```python
from build123d import *

# Parameters (mm, degrees)
SKETCH1_R           = 4.5
BOSS_EXTRUDE1_DEPTH = 5.5
SKETCH2_R           = 4.5
BOSS_EXTRUDE2_DEPTH = 6
SKETCH3_R           = 3
CUT_EXTRUDE1_DEPTH  = 5


with BuildPart() as part:
    # Sketch1 → Boss-Extrude1 (new body)
    with BuildSketch(Plane(origin=(0, 0, 0), x_dir=(1, 0, 0), z_dir=(0, 1, 0))):
        with Locations((-2.5, -1.5)):
            Circle(SKETCH1_R)
        with BuildLine():
            Line((-0.5, 0), (-4.5, 0))
            ThreePointArc((-4.5, 0), (-4.853553391, -0.146446609), (-5, -0.5))
            Line((-5, -0.5), (-5, -2.5))
            ThreePointArc((-5, -2.5), (-4.853553391, -2.853553391), (-4.5, -3))
            Line((-4.5, -3), (-0.5, -3))
            ThreePointArc((-0.5, -3), (-0.146446609, -2.853553391), (0, -2.5))
            Line((0, -2.5), (0, -0.5))
            ThreePointArc((0, -0.5), (-0.146446609, -0.146446609), (-0.5, 0))
        make_face(mode=Mode.SUBTRACT)
    extrude(amount=BOSS_EXTRUDE1_DEPTH)

    # Sketch2 → Boss-Extrude2 (add)
    with BuildSketch(Plane(origin=(0, 5.5, 0), x_dir=(1, 0, 0), z_dir=(0, 1, 0))):
        with Locations((-2.5, -1.5)):
            Circle(SKETCH2_R)
    extrude(amount=BOSS_EXTRUDE2_DEPTH)

    # Sketch3 → Cut-Extrude1 (cut)
    with BuildSketch(Plane(origin=(0, 11.5, 0), x_dir=(1, 0, 0), z_dir=(0, 1, 0))):
        with Locations((-2.5, -1.5)):
            Circle(SKETCH3_R)
    extrude(amount=-CUT_EXTRUDE1_DEPTH, mode=Mode.SUBTRACT)


solid = part.part
```
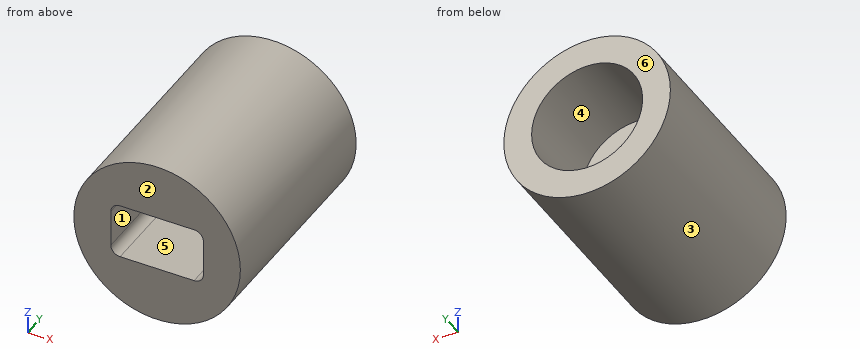
CAD build for the part. Positions are in the model's coordinates, mm. Face numbers are marked on the shaded views. A direction names the side the tool comes from. Round coordinates to 2 decimals unless told otherwise and drop trailing zeros. Write each loop counter-clockwise with the first axis right and the second up, starting at its lowest first coordinate (ties: lowest second). Pieces come first, ordered by that corner, then holes.
Item 1: Mould opens along Z. For the marked faces 1, 2 and 3 say: released by +Z, released by -Z, zero draft, split by the parting line, or undercut.
Filled in:
face 1: undercut
face 2: zero draft
face 3: split by the parting line
Item 2: Tool access for the marked faces 4, 5 and 6: list every direction of +Z, -Z, +X, -X, +Y, -Y with a clear straight run to the whole face (end or side of a thin tool).
Filled in:
face 4: +Y
face 5: -Y
face 6: +Z, -Z, +X, -X, +Y
Item 3: Band-saw the part on C-C on x = -2.5. Write the cut outline in (y, z), then the cut area to 3 significant figures.
Filled in:
outline: (0, -3) - (11.5, -3) - (11.5, -1.5) - (6.5, -1.5) - (6.5, 4.5) - (11.5, 4.5) - (11.5, 6) - (0, 6) - (0, 3) - (5.5, 3) - (5.5, 0) - (0, 0) - close
area: 57.0 mm2
Item 4: Band-saw the part on A-A on y = 1.25. Write the cut outline in (x, z), then the cut area to 3 significant figures.
Filled in:
outline: circle Ø9 at (-2.5, 1.5); hole (-5, 0.5) arc R0.5 ccw to (-4.5, 0) - (-0.5, 0) arc R0.5 ccw to (0, 0.5) - (0, 2.5) arc R0.5 ccw to (-0.5, 3) - (-4.5, 3) arc R0.5 ccw to (-5, 2.5) - close
area: 48.8 mm2
Item 5: Drill centre lines: L1, parallel to Z at x = -2.5, y = 7.65; L2, parallel to X at y = 7.5, z = 1.5; L3, parallel to Z at x = -2.5, y = 1.25. Where is each one in solid material? Low to high.
Filled in:
L1: z = -3 to -1.5, 4.5 to 6
L2: x = -7 to -5.5, 0.5 to 2
L3: z = -3 to 0, 3 to 6
Item 6: Drop flat-ended pins along their axis: pin 1 Ø1.5 at (x, z) = (-2.5, 1) entering from -Y; pin 2 Ø1.5 at (y, z) = (6.5, -1) entering from -X; pin 3 Ø4 at (x, y) = (0.5, 2) entering from -Z; pin 4 Ø2 at (x, y) = (-1.5, 7.5) entering from -Z. Give the stop position or say it passes through.
Filled in:
pin 1: stops at y = 5.5
pin 2: stops at x = -6.65
pin 3: stops at z = -2.89
pin 4: stops at z = -3
Item 7: Band-saw the part on D-D on x = -5.25. Write the cut outline in (y, z), then the cut area to 3 significant figures.
Filled in:
outline: (0, -2.06) - (11.5, -2.06) - (11.5, 0.3) - (6.5, 0.3) - (6.5, 2.7) - (11.5, 2.7) - (11.5, 5.06) - (0, 5.06) - close
area: 69.9 mm2
Item 8: Band-saw the part on B-B on z = 1.5. Write the cut outline in (x, y), then the cut area to 3 significant figures.
Filled in:
outline: (-7, 0) - (-5, 0) - (-5, 5.5) - (0, 5.5) - (0, 0) - (2, 0) - (2, 11.5) - (0.5, 11.5) - (0.5, 6.5) - (-5.5, 6.5) - (-5.5, 11.5) - (-7, 11.5) - close
area: 46.0 mm2
